from build123d import *

# Parameters (mm, degrees)
SKETCH2_R           = 1.905
BOSS_EXTRUDE1_DEPTH = 3.175
SKETCH3_W           = 12.7
SKETCH3_H           = 25.4
BOSS_EXTRUDE2_DEPTH = 1.5875
SKETCH5_R           = 1.905
BOSS_EXTRUDE3_DEPTH = 1.5875
FILLET1_R           = 2.54


with BuildPart() as part:
    # Sketch2 → Boss-Extrude1 (new, symmetric)
    with BuildSketch(Plane.XY):
        Circle(SKETCH2_R)
    extrude(amount=BOSS_EXTRUDE1_DEPTH, both=True)

    # Sketch3 → Boss-Extrude2 (add)
    with BuildSketch(Plane.XY.offset(3.175)):
        Rectangle(SKETCH3_W, SKETCH3_H)
    extrude(amount=BOSS_EXTRUDE2_DEPTH)

    # Sketch5 → Boss-Extrude3 (add, symmetric)
    with BuildSketch(Plane(origin=(0, 6.35, 0), x_dir=(1, 0, 0), z_dir=(0, 1, 0))):
        with BuildLine():
            Line((-3.175, -4.7625), (3.175, -4.7625))
            Line((3.175, -4.7625), (3.175, -11.1125))
            ThreePointArc((3.175, -11.1125), (0, -14.2875), (-3.175, -11.1125))
            Line((-3.175, -11.1125), (-3.175, -4.7625))
        make_face()
        with Locations(Location((0, -11.1125, 0), (0, 0, 270))):
            Circle(SKETCH5_R, mode=Mode.SUBTRACT)
    boss_extrude3 = extrude(amount=BOSS_EXTRUDE3_DEPTH, both=True)

    # Mirror1: Boss-Extrude3 across plane
    add(boss_extrude3.mirror(Plane.ZX))

    # Fillet1
    fillet1_edges = [part.edges().sort_by_distance(p)[0] for p in [
        (6.35, -12.7, 3.96875),
        (6.35, 12.7, 3.96875),
        (-6.35, 12.7, 3.96875),
        (-6.35, -12.7, 3.96875),
    ]]
    fillet(fillet1_edges, radius=FILLET1_R)


solid = part.part
Could you check a few things on this model? Use its own coordinates, in mm. A direction names the side the tool comes from. Coordinates: 2 decimals unless noted, no trailing zeros. Write each loop counter-clockwise with the first axis right and the second up, starting at its lowest first coordinate (ties: lowest second). Pieces come first, ordered by that corner, then holes. Notation, with made-up numbers: (81, 82) - (101, 82) arc R16 cw to (101, 96) - close; hole circle Ø8 at (69, 48). An arc over 180 degrees is marked (long way). Write item = value, one per line.
1) Will these pins go through, and if not, where does the flat tip stop? pin 1 Ø7 at (x, z) = (-1, 11) entering from -Y; pin 2 Ø6 at (y, z) = (-6, 3) entering from +X; pin 3 Ø2.5 at (y, z) = (7, 9.5) entering from -X (3 decimals); pin 4 Ø1 at (x, y) = (1.5, 7.5) entering from -Z (3 decimals).
Result set:
pin_1 = -7.94
pin_2 = 6.35
pin_3 = -3.175
pin_4 = 3.175
2) Suppose I cut it at A-A on x = 0. Please give me the cut outline in (y, z) (1 decimal).
Result set:
outline = (-12.7, 3.2) - (-1.9, 3.2) - (-1.9, -3.2) - (1.9, -3.2) - (1.9, 3.2) - (12.7, 3.2) - (12.7, 4.8) - (7.9, 4.8) - (7.9, 9.2) - (4.8, 9.2) - (4.8, 4.8) - (-4.8, 4.8) - (-4.8, 9.2) - (-7.9, 9.2) - (-7.9, 4.8) - (-12.7, 4.8) - close; (-7.9, 13) - (-4.8, 13) - (-4.8, 14.3) - (-7.9, 14.3) - close; (4.8, 13) - (7.9, 13) - (7.9, 14.3) - (4.8, 14.3) - close
3) Please list where these lines run through material, in increasing order: line 1 (Y direction, x = -1.5, z = 9.75); line 2 (Z direction, x = 2.5, y = -3) (1 decimal); line 3 (X direction, y = -5, z = 11.5). Write a range as [from, to].
Result set:
line_1 = [-7.94, -4.76], [4.76, 7.94]
line_2 = [3.2, 4.8]
line_3 = [-3.15, -1.87], [1.87, 3.15]
4) Suppose I cut it at C-C on z = 12.75. Please give me the cut outline in (x, y), plus the area to 3 significant figures.
Result set:
outline = (-2.72, -7.94) - (-0.97, -7.94) - (-0.97, -4.76) - (-2.72, -4.76) - close; (-2.72, 4.76) - (-0.97, 4.76) - (-0.97, 7.94) - (-2.72, 7.94) - close; (0.97, -7.94) - (2.72, -7.94) - (2.72, -4.76) - (0.97, -4.76) - close; (0.97, 4.76) - (2.72, 4.76) - (2.72, 7.94) - (0.97, 7.94) - close
area = 22.2 mm2
5) For faces 1 (the cylindrical face through (5.586, 11.976, 3.98)), 2 (the cylindrical face through (0.07, -6.372, 14.287)), 3 (the cylindrical face through (-0.41, -1.86, 0.04)), 4 (the flat face through (-3.175, -6, 8)), 5 (the flat face through (0, -4.762, 8)), which set-ups out of +Z, -Z, +X, -X, +Y, -Y let a thin tool reach every point of the face, with its end or its side?
Result set:
face_1 = +Z, -Z, +X, +Y
face_2 = +Z, +Y, -Y
face_3 = -Z
face_4 = +Z, -X, +Y, -Y
face_5 = +Z, +X, -X
6) We'd pull the mould along X, two halves only. Please class faces 6 (the cylindrical face through (0.08, -6.33, 9.21)), 7 (the flat face through (0, 7.938, 8)), 8 (the cylindrical face through (5.586, -11.976, 3.98)), 9 (the cylindrical face through (0.08, 6.33, 9.21)): +X half, -X half, draft (parallel to the pull), parting line (faces both ways), or undercut.
Result set:
face_6 = undercut
face_7 = draft
face_8 = +X half
face_9 = undercut
